Check sheet for the modelled part. Datum: model origin and axes. Units: mm. A direction names the side the tool comes from. Give positions to 0.01 mm unless a question says otherwise; leave off trailing zeros. Loops run counter-clockwise (first coordinate to the right, second up) from the corner with the lowest first, then second, coordinate; pieces in that order, holes last. Notation, with made-up numbers: M 10.5,7 L 16.5,7 A19 cw 16.5,15 Z; hole C 34.5,85 d8. An arc over 180 degrees is marked long. One line per question, with ' | ' between items. Start each with the question number.
from build123d import *

# Parameters (mm, degrees)
F0_W      = 28
F0_H      = 60
F4_DEPTH  = 3
F2_W      = 28
F2_H      = 7.8
F5_DEPTH  = 7.8
F3_W      = 28
F3_H      = 12.2
F6_DEPTH  = 7
F7_R      = 0.8
F8_DEPTH  = 25
F9_R      = 0.8
F10_DEPTH = 25
F11_R     = 1.25
F13_DEPTH = 25
F12_R     = 1.25
F14_DEPTH = 25
F15_SIZE  = 0.5
F16_R     = 1.25
F17_DEPTH = 25


with BuildPart() as f4:
    # F0 (on Top) → F4 (new body)
    with BuildSketch(Plane.XY):
        with Locations((14, 30)):
            Rectangle(F0_W, F0_H)
    extrude(amount=F4_DEPTH)

    # F2 (on face) → F5 (join)
    with BuildSketch(Plane.XY):
        with Locations((14, 12.1)):
            Rectangle(F2_W, F2_H)
    extrude(amount=F5_DEPTH)

    # F3 (on face) → F6 (join)
    with BuildSketch(Plane.XY):
        with Locations((14, 22.1)):
            Rectangle(F3_W, F3_H)
    extrude(amount=F6_DEPTH)

    # F7 (on face) → F8 (cut)
    with BuildSketch(Plane.XY.offset(3)):
        with Locations((6, 53.5)):
            Circle(F7_R)
    extrude(amount=-F8_DEPTH, mode=Mode.SUBTRACT)

    # F9 (on face) → F10 (cut)
    with BuildSketch(Plane.XY.offset(3)):
        with Locations((22, 53.5)):
            Circle(F9_R)
    extrude(amount=-F10_DEPTH, mode=Mode.SUBTRACT)

    # F11 (on face) → F13 (cut)
    with BuildSketch(Plane.XY.offset(3)):
        with Locations((6, 4)):
            Circle(F11_R)
    extrude(amount=-F13_DEPTH, mode=Mode.SUBTRACT)

    # F12 (on face) → F14 (cut)
    with BuildSketch(Plane.XY.offset(3)):
        with Locations((22, 4)):
            Circle(F12_R)
    extrude(amount=-F14_DEPTH, mode=Mode.SUBTRACT)

    # F15
    f15_edges = [f4.edges().sort_by_distance(p)[0] for p in [
        (28, 0, 1.5),
        (0, 0, 1.5),
        (0, 60, 1.5),
        (28, 60, 1.5),
    ]]
    chamfer(f15_edges, length=F15_SIZE)

    # F16 (on face) → F17 (cut)
    with BuildSketch(Plane.XY.offset(7)):
        with Locations((24, 22.2)):
            Circle(F16_R)
    extrude(amount=-F17_DEPTH, mode=Mode.SUBTRACT)


solid = f4.part
Q1. Draft check along X on faces 4 (the flat face through (0, 23, 3)), 5 (the cylindrical face through (23.155, 3.521, 1.521)), 6 (the flat face through (14, 60, 1)). Enter one of: released by +X, released by -X, zero draft, split by the parting line, or undercut.
Q2. Cross-section at D-D (x = 3.75). Record the cut outline in (y, z), and give its area (3 significant figures).
Q3. Cross-section at C-C (y = 22.2). Record the cut outline in (x, z).
Q4. Material ranges on probe 1 along Y at (x, z) = (6, 1); probe 2 along Y at (x, z) = (24, 2.5); probe 3 along Y at (x, z) = (20.25, 5), recorded low to high. Write a range as from..to.
Q5. Depth check by flat-ended pin: P1, Ø2.5, axis at x = 9.5, y = 4, coming from the +Z side; P2, Ø0.9, axis at x = 16, z = 7.5, coming from the +Y side; P3, Ø3, axis at x = 3.5, z = 5.5, coming from the +Y side. Enter the tip coordinate at first touch or a pass-through.
Q6. Access from +Z, -Z, +X, -X, +Y, -Y to the whole of each face (thin tool, end or side, straight path). Record for faces 1 (the flat face through (14, 28.2, 5)), 2 (the flat face through (14, 8.2, 5)), 3 (the flat face through (14, 30, 0)).
Q7. Cross-section at A-A (x = 22). Record the cut outline in (y, z), and give its area (3 significant figures).
Q8. Cross-section at B-B (y = 4). Record the cut outline in (x, z), and give its area (3 significant figures).
Solved:
1) face 4: released by -X | face 5: undercut | face 6: zero draft
2) outline: M 0,0 L 60,0 L 60,3 L 28.2,3 L 28.2,7 L 16,7 L 16,7.8 L 8.2,7.8 L 8.2,3 L 0,3 Z | area: 266 mm²
3) outline: M 0,0 L 22.75,0 L 22.75,7 L 0,7 Z; M 25.25,0 L 28,0 L 28,7 L 25.25,7 Z
4) probe 1: y = 0..2.75, 5.25..52.7, 54.3..60 | probe 2: y = 0..20.95, 23.45..60 | probe 3: y = 8.2..28.2
5) P1: stops at z = 3 | P2: stops at y = 16 | P3: stops at y = 28.2
6) face 1: +Z, +X, -X, +Y | face 2: +Z, +X, -X, -Y | face 3: -Z, +X, -X, +Y, -Y
7) outline: M 0,0 L 2.75,0 L 2.75,3 L 0,3 Z; M 5.25,0 L 52.7,0 L 52.7,3 L 28.2,3 L 28.2,7 L 16,7 L 16,7.8 L 8.2,7.8 L 8.2,3 L 5.25,3 Z; M 54.3,0 L 60,0 L 60,3 L 54.3,3 Z | area: 254 mm²
8) outline: M 0,0 L 4.75,0 L 4.75,3 L 0,3 Z; M 7.25,0 L 20.75,0 L 20.75,3 L 7.25,3 Z; M 23.25,0 L 28,0 L 28,3 L 23.25,3 Z | area: 69.0 mm²
